Answer from the drawing. Dimensions are ordinates in mm from the lowest x, y and z of the part. A direction names the side the tool comes from. Give positions to 0.01 mm unless a question says otherwise; leave off trailing zeros. Order: outer loops, then holes, each group sorted by start corner. A loop starts at its lowest first (then second) coordinate and runs counter-clockwise, first axis right, second up. Notation, with made-up numbers: (45.25, 1) - (95.25, 1) arc R21 cw to (95.25, 33) - close; hole circle Ø6 at (69, 3). An arc over 180 degrees is marked (long way). Answer in a Markdown table with one row per item.
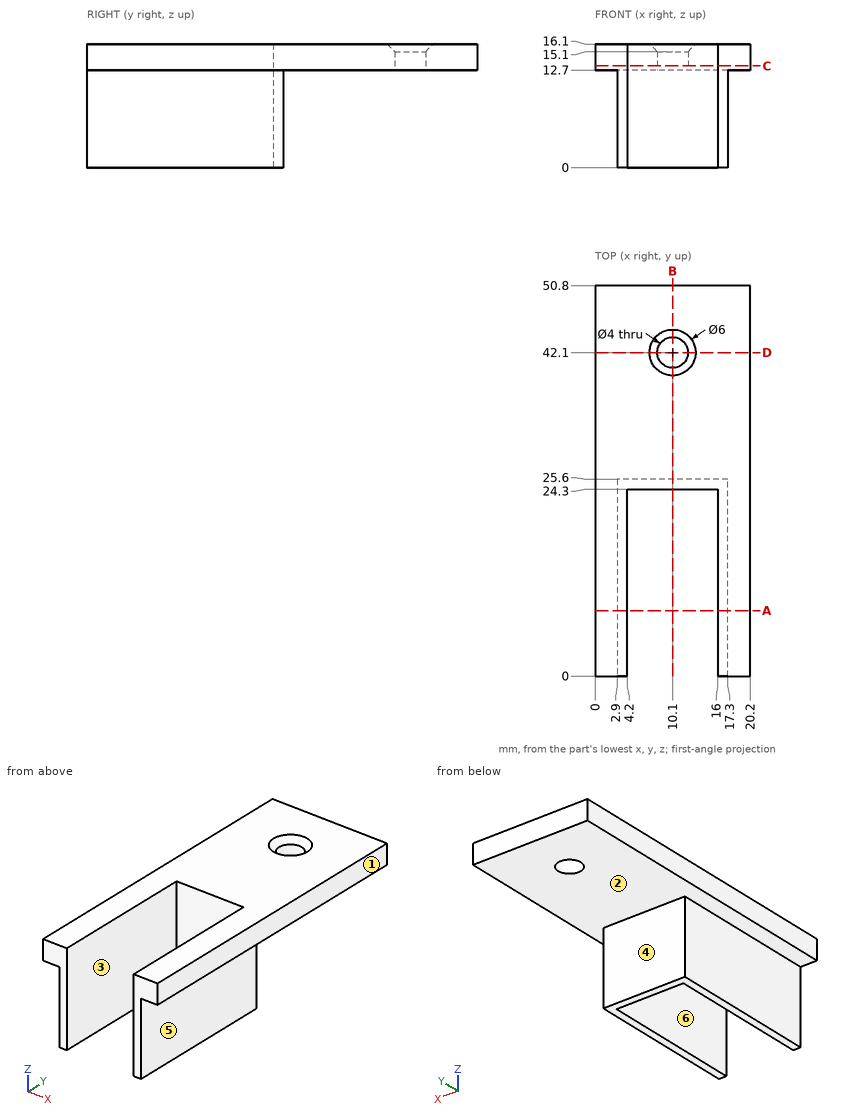
Item 1: Determine the mould class of the marked faces 1, 2 and 3 for opening direction X: pulls with the +X half, pulls with the -X half, needs draft (parallel to the pull), parting line crosses it, or undercut.
Answer block:
| item | result |
|---|---|
| face 1 | pulls with the +X half |
| face 2 | needs draft |
| face 3 | undercut |
Item 2: Which of the six approach directions +Z, -Z, +X, -X, +Y, -Y give full straight-line access (tool end or side, diameter ignored) to the marked faces 4, 5 and 6?
Answer block:
| item | result |
|---|---|
| face 4 | -Z, +X, -X, +Y |
| face 5 | -Z, +X, +Y, -Y |
| face 6 | +Z, -Z, -Y |
Item 3: Find section D-D on y = 42.1. Write down the section's boundary in (x, z), then the cut area to 3 significant figures.
Answer block:
| item | result |
|---|---|
| outline | (0, 12.7) - (8.1, 12.7) - (8.1, 15.1) - (7.1, 16.1) - (0, 16.1) - close; (12.1, 12.7) - (20.2, 12.7) - (20.2, 16.1) - (13.1, 16.1) - (12.1, 15.1) - close |
| area | 54.1 mm² |
Item 4: Find section B-B on x = 10.1. Write down the section's boundary in (y, z), then the cut area to 3 significant figures.
Answer block:
| item | result |
|---|---|
| outline | (24.3, 0) - (25.6, 0) - (25.6, 12.7) - (40.1, 12.7) - (40.1, 15.1) - (39.1, 16.1) - (24.3, 16.1) - close; (44.1, 12.7) - (50.8, 12.7) - (50.8, 16.1) - (45.1, 16.1) - (44.1, 15.1) - close |
| area | 92.0 mm² |
Item 5: Consider line 1 (Y direction, x = 10.1, z = 14); line 2 (X direction, y = 42.1, z = 13.8); line 3 (Z direction, x = 6.25, y = 46.5). Determine where each line is inside the solid, lowest interval first.
Answer block:
| item | result |
|---|---|
| line 1 | 24.3 to 40.1, 44.1 to 50.8 |
| line 2 | 0 to 8.1, 12.1 to 20.2 |
| line 3 | 12.7 to 16.1 |
Item 6: Find section C-C on z = 13.25. Write down the section's boundary in (x, y), then the cut area to 3 significant figures.
Answer block:
| item | result |
|---|---|
| outline | (0, 0) - (4.2, 0) - (4.2, 24.3) - (16, 24.3) - (16, 0) - (20.2, 0) - (20.2, 50.8) - (0, 50.8) - close; hole circle Ø4 at (10.1, 42.1) |
| area | 727 mm² |
Item 7: Find section A-A on y = 8.5. Write down the section's boundary in (x, z), then the cut area to 3 significant figures.
Answer block:
| item | result |
|---|---|
| outline | (0, 12.7) - (2.9, 12.7) - (2.9, 0) - (4.2, 0) - (4.2, 16.1) - (0, 16.1) - close; (16, 0) - (17.3, 0) - (17.3, 12.7) - (20.2, 12.7) - (20.2, 16.1) - (16, 16.1) - close |
| area | 61.6 mm² |
Item 8: Each of these flat-tipped pins is pushed along its axis until it touches: P1, Ø8, axis at x = 16, y = 42, coming from the -Z side; P2, Ø5, axis at y = 14, z = 5.5, coming from the -X side; P3, Ø5, axis at y = 12, z = 10, coming from the +X side. Where does it stop, or does it pass through?
Answer block:
| item | result |
|---|---|
| P1 | z = 12.7 |
| P2 | x = 2.9 |
| P3 | x = 17.3 |
